The model under review builds one solid part; all positions refer to its coordinate system, in mm. Face numbers are marked on the shaded views. Coordinates: 2 decimals unless noted, no trailing zeros. Write each loop counter-clockwise with the first axis right and the second up, starting at its lowest first coordinate (ties: lowest second). Pieces come first, ordered by that corner, then holes. Notation, with made-up numbers: (78, -22) - (111, -22) arc R26 ccw to (111, -4) - close; hole circle Ø10 at (38, 6.25). An arc over 180 degrees is marked (long way). Answer as CSV lines item,"result". Start each with the question number.
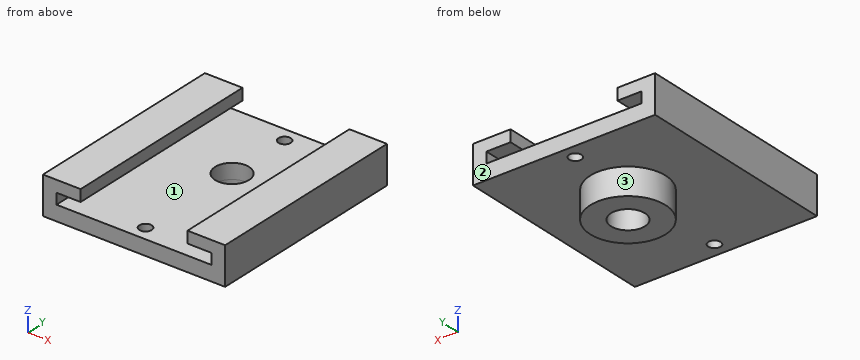
```python
from build123d import *

# Parameters (mm, degrees)
F0_W     = 34.0868
F0_H     = 38.481
F1_DEPTH = 7.0358
F2_W     = 20.0152
F2_H     = 2.1844
F3_DEPTH = 38.482
F4_W     = 29.0322
F4_H     = 2.032
F5_DEPTH = 38.482
F6_R     = 1.1557
F6_R_2   = 3.175
F7_DEPTH = 25.4
F8_R     = 7.0485
F8_R_2   = 3.175
F9_DEPTH = 5.0038


with BuildPart() as f1:
    # F0 (on Top) → F1 (new body)
    with BuildSketch(Plane.XY):
        with Locations((-27.354376, 30.454514)):
            Rectangle(F0_W, F0_H)
    extrude(amount=F1_DEPTH)

    # F2 (on face) → F3 (cut, through all)
    with BuildSketch(Plane.XZ.offset(-11.214014)):
        with Locations((-27.354376, 5.9436)):
            Rectangle(F2_W, F2_H)
    extrude(amount=-F3_DEPTH, mode=Mode.SUBTRACT)

    # F4 (on face) → F5 (cut, through all)
    with BuildSketch(Plane.XZ.offset(-11.214014)):
        with Locations((-27.354376, 3.8354)):
            Rectangle(F4_W, F4_H)
    extrude(amount=-F5_DEPTH, mode=Mode.SUBTRACT)

    # F6 (on face) → F7 (cut)
    with BuildSketch(Plane(origin=(0, 0, 0), x_dir=(1, 0, 0), z_dir=(0, 0, -1))):
        with Locations((-27.354376, -13.944514)):
            Circle(F6_R)
        with Locations((-27.354376, -34.505814)):
            Circle(F6_R_2)
        with Locations((-27.354376, -47.015314)):
            Circle(F6_R)
    extrude(amount=-F7_DEPTH, mode=Mode.SUBTRACT)

    # F8 (on face) → F9 (join)
    with BuildSketch(Plane(origin=(0, 0, 0), x_dir=(1, 0, 0), z_dir=(0, 0, -1))):
        with Locations((-27.354376, -34.505814)):
            Circle(F8_R)
        with Locations((-27.354376, -34.505814)):
            Circle(F8_R_2, mode=Mode.SUBTRACT)
    extrude(amount=F9_DEPTH)


solid = f1.part
```
(1) Add section D-D on y = 20. Give the boundary of the cut face in (x, z), then the cut area to 3 significant figures.
(2) For pin 1 (14.5 mm diameter, centred on x = -26, y = 33.5, fed in from +Z); pin 2 (4 mm diameter, centred on x = -28.5, y = 21.5, fed in from -Z); pin 3 (5 mm diameter, centred on x = -27.35, y = 34.51, fed in from +Z), all flat-tipped, find the tip position at first contact; note any pin that passes through.
(3) Add section B-B on z = 5.5. Give the boundary of the cut face in (x, y).
(4) Add section C-C on y = 34. Give the boundary of the cut face in (x, z).
(5) The part is to be moulded in two halves that separate along X. For the marked faces 1, 2 and 3, say which applies: released by +X, released by -X, zero draft, split by the parting line, or undercut.
(6) Add section A-A on x = -41. Give the boundary of the cut face in (y, z), then the cut area to 3 significant figures.
(7) Wall thickness on line 1 (X direction, y = 15.5, z = 3); line 2 (X direction, y = 17.5, z = 5.75); line 3 (Z direction, x = -13, y = 34): over which ranges is each line inside the solid? List them lowest first.
Reported:
1,outline,"(-44.4, 0) - (-10.31, 0) - (-10.31, 7.04) - (-17.35, 7.04) - (-17.35, 4.85) - (-12.84, 4.85) - (-12.84, 2.82) - (-41.87, 2.82) - (-41.87, 4.85) - (-37.36, 4.85) - (-37.36, 7.04) - (-44.4, 7.04) - close"
1,area,"137 mm²"
2,pin 1,"z = 2.82"
2,pin 2,"z = 0"
2,pin 3,"through"
3,outline,"(-44.4, 11.21) - (-37.36, 11.21) - (-37.36, 49.7) - (-44.4, 49.7) - close; (-17.35, 11.21) - (-10.31, 11.21) - (-10.31, 49.7) - (-17.35, 49.7) - close"
4,outline,"(-44.4, 0) - (-34.38, 0) - (-34.38, -5) - (-30.49, -5) - (-30.49, 2.82) - (-41.87, 2.82) - (-41.87, 4.85) - (-37.36, 4.85) - (-37.36, 7.04) - (-44.4, 7.04) - close; (-24.22, -5) - (-20.32, -5) - (-20.32, 0) - (-10.31, 0) - (-10.31, 7.04) - (-17.35, 7.04) - (-17.35, 4.85) - (-12.84, 4.85) - (-12.84, 2.82) - (-24.22, 2.82) - close"
5,face 1,"undercut"
5,face 2,"zero draft"
5,face 3,"split by the parting line"
6,outline,"(11.21, 0) - (49.7, 0) - (49.7, 2.82) - (11.21, 2.82) - close; (11.21, 4.85) - (49.7, 4.85) - (49.7, 7.04) - (11.21, 7.04) - close"
6,area,"193 mm²"
7,line 1,"-44.4 to -41.87, -12.84 to -10.31"
7,line 2,"-44.4 to -37.36, -17.35 to -10.31"
7,line 3,"0 to 2.82, 4.85 to 7.04"
